```python
from build123d import *

# Parameters (mm, degrees)
F0_R     = 19.05
F0_R_2   = 6.35
F1_DEPTH = 12.7
F2_R     = 5.08
F3_DEPTH = 12.7
F4_R     = 5.08


with BuildPart() as f1:
    # F0 (on Top) → F1 (new body, symmetric)
    with BuildSketch(Plane.XY):
        Circle(F0_R)
        Circle(F0_R_2, mode=Mode.SUBTRACT)
    extrude(amount=F1_DEPTH, both=True)

    # F2
    f2_edges = [f1.edges().sort_by_distance(p)[0] for p in [
        (-19.05, 0, -12.7),
        (-19.05, 0, 12.7),
    ]]
    fillet(f2_edges, radius=F2_R)

    # F0 (on Top) → F3 (join, symmetric)
    with BuildSketch(Plane.XY):
        Circle(F0_R)
        Circle(F0_R_2, mode=Mode.SUBTRACT)
    extrude(amount=F3_DEPTH, both=True)

    # F4
    f4_edges = [f1.edges().sort_by_distance(p)[0] for p in [
        (-19.05, 0, -12.7),
        (-19.05, 0, 12.7),
    ]]
    fillet(f4_edges, radius=F4_R)


solid = f1.part
```
The model under review builds one solid part; all positions refer to its coordinate system, in mm. Coordinates: 2 decimals unless noted, no trailing zeros. Write each loop counter-clockwise with the first axis right and the second up, starting at its lowest first coordinate (ties: lowest second). Pieces come first, ordered by that corner, then holes.
1) The part is to be moulded in two halves that separate along Y. For faces 1 (the face through (-15.12, -11.59, 0.11)), 2 (the face through (6, -3, 12.7)), 3 (the face through (-1.38, -6.2, -0.18)), say which applies: pulls with the +Y half, pulls with the -Y half, needs draft (parallel to the pull), parting line crosses it, or undercut.
2) We need section D-D on z = -10.5. State the section outline as (x, y) points, then the cut area to 3 significant figures.
3) We need section C-C on z = 6.5. State the section outline as (x, y) points.
4) To check wall thickness, follow probe 1 along Y at (x, z) = (0, -7); probe 2 along Z at (x, y) = (13, 5.5); probe 3 along X at (y, z) = (1, -10.75). State the ranges of each line that lie inside material, in increasing order.
5) We need section A-A on x = 0. State the section outline as (y, z) points.
6) Clearance check with flat-ended pins moving along their axes: pin 1 Ø5 at (y, z) = (-12, 7.5) entering from -X; pin 2 Ø7.5 at (x, y) = (0, 0) entering from +Z; pin 3 Ø12 at (x, y) = (-9.5, 14) entering from +Z; pin 4 Ø8 at (x, z) = (-11.5, 9) entering from -Y. State where each tip first meets the part, or that it passes through.
Answer list:
1. face 1: parting line crosses it
1. face 2: needs draft
1. face 3: undercut
2. outline: circle Ø36.31 at (0, 0); hole circle Ø12.7 at (0, 0)
2. area: 909 mm2
3. outline: circle Ø38.1 at (0, 0); hole circle Ø12.7 at (0, 0)
4. probe 1: y = -19.05 to -6.35, 6.35 to 19.05
4. probe 2: z = -12.7 to 12.7
4. probe 3: x = -17.94 to -6.27, 6.27 to 17.94
5. outline: (-19.05, -7.62) arc R5.08 ccw to (-13.97, -12.7) - (-6.35, -12.7) - (-6.35, 12.7) - (-13.97, 12.7) arc R5.08 ccw to (-19.05, 7.62) - close; (6.35, -12.7) - (13.97, -12.7) arc R5.08 ccw to (19.05, -7.62) - (19.05, 7.62) arc R5.08 ccw to (13.97, 12.7) - (6.35, 12.7) - close
6. pin 1: stops at x = -16.51
6. pin 2: passes through
6. pin 3: stops at z = 12.7
6. pin 4: stops at y = -17.44
